Part model, mm, in its own coordinate system. A direction names the side the tool comes from. Round coordinates to 2 decimals unless told otherwise and drop trailing zeros. Write each loop counter-clockwise with the first axis right and the second up, starting at its lowest first coordinate (ties: lowest second). Pieces come first, ordered by that corner, then holes.
from build123d import *

# Parameters (mm, degrees)
BASEHEAD_DEPTH  = 13.3096
THDSCHPAT_COUNT = 12
THDSCHPAT_PITCH = 2.434166667


with BuildPart() as part:
    # Sketch1 → BaseHead (new body)
    with BuildSketch(Plane(origin=(0, 0, 0), x_dir=(0, 0, -1), z_dir=(1, 0, 0))):
        Polygon((14.2875, 8.248891971), (14.2875, -8.248891971), (0, -16.497783942), (-14.2875, -8.248891971), (-14.2875, 8.248891971), (0, 16.497783942), align=None)
    extrude(amount=BASEHEAD_DEPTH)

    # BodySke → BaseBody (revolve)
    with BuildSketch(Plane.XY, mode=Mode.PRIVATE) as basebody_sk:
        Polygon((0, 0), (45.0596, 0), (45.0596, 8.01243), (43.54703, 9.525), (0, 9.525), align=None)
    revolve(basebody_sk.sketch.rotate(Axis((0, 0, 0), (1, 0, 0)), 90), axis=Axis((0, 0, 0), (1, 0, 0)))

    # Sketch3 → HeadChamfer (revolve, cut)
    with BuildSketch(Plane.XY):
        Polygon((0, 14.2875), (4.942282238, 22.847783942), (4.942282238, 29.197783942), (-12.7, 29.197783942), (-12.7, 14.2875), align=None)
    revolve(axis=Axis((0, 0, 0), (1, 0, 0)), mode=Mode.SUBTRACT)

    # ThdSchSke → ThreadSchematic (revolve, cut)
    with BuildSketch(Plane.XY):
        Polygon((15.8496, -8.01243), (14.790487084, -9.525), (14.790487084, -11.90625), (16.908712916, -11.90625), (16.908712916, -9.525), align=None)
    threadschematic = revolve(axis=Axis((-3.175, 0, 0), (1, 0, 0)), mode=Mode.SUBTRACT)

    # ThdSchPat: ThreadSchematic ×12
    with Locations(*[(i * THDSCHPAT_PITCH, 0, 0) for i in range(1, THDSCHPAT_COUNT)]):
        add(threadschematic, mode=Mode.SUBTRACT)


solid = part.part
Q1. Tool access for faces 1 (the conical face through (0.31, 7.44, 12.82)), 2 (the cylindrical face through (24.37, 3.65, 8.8)): list every direction of +Z, -Z, +X, -X, +Y, -Y with a clear straight run to the whole face (end or side of a thin tool).
Q2. Drop flat-ended pins along their axis: P1, Ø4, axis at y = 13, z = 0.5, coming from the +X side; P2, Ø6, axis at x = 30, z = -0.5, coming from the +Y side (3 decimals); P3, Ø1.5, axis at x = 27.5, y = 4.5, coming from the +Z side. Give the stop position or say it passes through.
Q3. Two-plate mould, pull along X, no slides. Class faces 3 (the cylindrical face through (34.1, 3.65, 8.8)), 4 (the conical face through (0.31, 7.38, -12.86)): released by +X, released by -X, zero draft, split by the parting line, or undercut.
Q4. Wall check: line 1 (X direction, y = -5.5, z = 9.75); line 2 (Z direction, x = 32, y = -5.5); line 3 (Y direction, x = 32.5, z = 6.5). Give the ranges that are in metal, low to high.
Q5. Saw through at A-A, the plane x = 11.5. Write the cut outline in (y, z).
Computed:
1. face 1: +Z, -X, +Y
1. face 2: +X
2. P1: stops at x = 13.31
2. P2: stops at y = 9.525
2. P3: stops at z = 8.65
3. face 3: zero draft
3. face 4: released by -X
4. line 1: x = 0 to 13.31
4. line 2: z = -7.48 to 7.48
4. line 3: y = -5.58 to 5.58
5. outline: (-16.5, 0) - (-8.25, -14.29) - (8.25, -14.29) - (16.5, 0) - (8.25, 14.29) - (-8.25, 14.29) - close
